```python
from build123d import *

# Parameters (mm, degrees)
F1_DEPTH = 6.35
F2_DEPTH = 6.35


with BuildPart() as f1:
    # F0 (on Top) → F1 (new body)
    with BuildSketch(Plane.XY):
        Polygon((6.785307, 32.889859), (6.973788, 23.842792), (6.785307, 9.141308), (6.973781, 0), (18.656539, 0.240873), (18.232433, 20.810728), (24.50015, 20.939954), (38.073074, 0), (51.266711, 0), (34.491945, 24.408581), (36.942191, 25.162537), (40.711805, 28.178345), (43.727491, 32.513574), (44.669896, 35.906363), (44.669896, 41.561004), (42.785086, 47.592629), (38.261559, 51.55088), (31.099292, 54.566693), (24.313992, 55.132158), (16.774772, 55.132158), (6.7853, 54.755177), (6.565141, 45.518056), align=None)
        Polygon((18.471096, 30.628692), (18.471096, 45.519255), (24.502473, 45.707747), (28.272083, 44.765305), (31.853214, 42.880423), (32.9841, 39.676126), (32.9841, 36.283337), (31.099292, 33.079039), (28.460566, 31.382646), (24.125513, 30.628692), align=None, mode=Mode.SUBTRACT)
    extrude(amount=F1_DEPTH)

    # F0 (on Top) → F2 (join)
    with BuildSketch(Plane.XY):
        Polygon((-10.177946, 19.69622), (-8.293139, 21.581025), (-5.654412, 23.277351), (-2.261762, 23.842792), (6.973788, 23.842792), (6.785307, 32.889859), (-0.942398, 33.07834), (-5.46593, 34.020742), (-8.293139, 36.470992), (-9.047061, 38.355795), (-8.858582, 41.748447), (-6.785294, 44.387174), (-2.450243, 45.518057), (0.376968, 45.518057), (6.565141, 45.518056), (6.7853, 54.755177), (2.450247, 54.755177), (-9.424023, 54.376644), (-15.643883, 52.114875), (-18.471091, 49.85311), (-20.732858, 45.518057), (-21.109819, 38.921238), (-19.413493, 33.832264), (-16.020843, 30.251132), (-12.816672, 29.308728), (-15.266922, 28.366325), (-18.659571, 26.293041), (-20.544375, 24.219753), (-21.67526, 21.204065), (-22.806143, 16.86901), (-21.863741, 11.591555), (-20.732858, 7.821944), (-18.471091, 4.806255), (-15.643883, 2.732969), (-11.49731, 1.225124), (-6.219853, -0.376961), (6.973781, 0), (6.785307, 9.141308), (-0.942398, 8.952827), (-4.71201, 9.70675), (-9.047061, 11.780035), (-10.177946, 14.418763), (-10.177946, 17.057493), align=None)
    extrude(amount=F2_DEPTH)


solid = f1.part
```
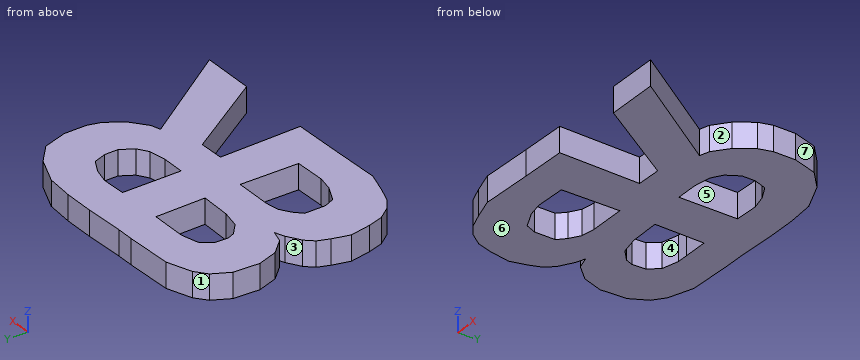
CAD build for the part. Positions are in the model's coordinates, mm. Face numbers are marked on the shaded views. A direction names the side the tool comes from. Round coordinates to 2 decimals unless told otherwise and drop trailing zeros. Write each loop counter-clockwise with the first axis right and the second up, starting at its lowest first coordinate (ties: lowest second). Pieces come first, ordered by that corner, then holes. Notation, with made-up numbers: M -18.75,74 L 12.25,74 A15 cw 12.25,81 Z; hole C 78,7 d5. An arc over 180 degrees is marked long. One line per question, with ' | ' between items.
1. Which spindle directions (+Z, -Z, +X, -X, +Y, -Y) get a long thin tool onto all of the face, cutting with end or side? Do the marked faces 1, 2, 3 and 4. Say none if no direction does.
Working result:
face 1: +Z, -Z, -X, +Y | face 2: +Z, -Z, +X | face 3: +Z, -Z, -X | face 4: +Z, -Z
2. Probe L1, parallel to Y at x = 0, z = 1; L2, parallel to Y at x = -4.5, z = 2.25; L3, parallel to X at y = 16.5, z = 1.75. List the from-to ranges inside material, lowest first. Write a range as from..to.
Working result:
L1: -0.2..8.98, 23.84..33.06, 45.52..54.68 | L2: -0.33..9.66, 23.47..33.82, 44.98..54.53 | L3: -22.74..-10.18, 6.88..18.32, 27.38..39.93
3. Pin check, flat tips, straight feed: pin 1 Ø1.6 at (y, z) = (17.5, 2) entering from +X; pin 2 Ø2 at (y, z) = (36.5, 5.5) entering from -X; pin 3 Ø1 at (y, z) = (23, 5.5) entering from +X. Stop position of each tip, or through.
Working result:
pin 1: x = 39.79 | pin 2: x = -20.64 | pin 3: x = 35.8
4. Mould opens along Y. For the marked faces 5, 6 and 7 say: pulls with the +Y half, pulls with the -Y half, needs draft (parallel to the pull), parting line crosses it, or undercut.
Working result:
face 5: undercut | face 6: needs draft | face 7: pulls with the +Y half
5. Cut at D-D on x = 46. Write the cut outline in (y, z), and give its area (3 significant figures).
Working result:
outline: M 0,0 L 7.66,0 L 7.66,6.35 L 0,6.35 Z | area: 48.7 mm2
6. Cut at A-A on x = 27.5. Write the cut outline in (y, z), and give its area (3 significant figures).
Working result:
outline: M 16.31,0 L 31.22,0 L 31.22,6.35 L 16.31,6.35 Z; M 44.96,0 L 54.87,0 L 54.87,6.35 L 44.96,6.35 Z | area: 158 mm2
7. Cut at C-C on y = 49. Write the cut outline in (x, z), and give its area (3 significant figures).
Working result:
outline: M -18.92,0 L 41.18,0 L 41.18,6.35 L -18.92,6.35 Z | area: 382 mm2
8. Cut at B-B on z = 1.5. Count the separate pieces of the cut face and the enclosed holes in it, and give its area (3 significant figures).
Working result:
separate pieces: 1 | enclosed holes: 3 | area: 2,500 mm2
